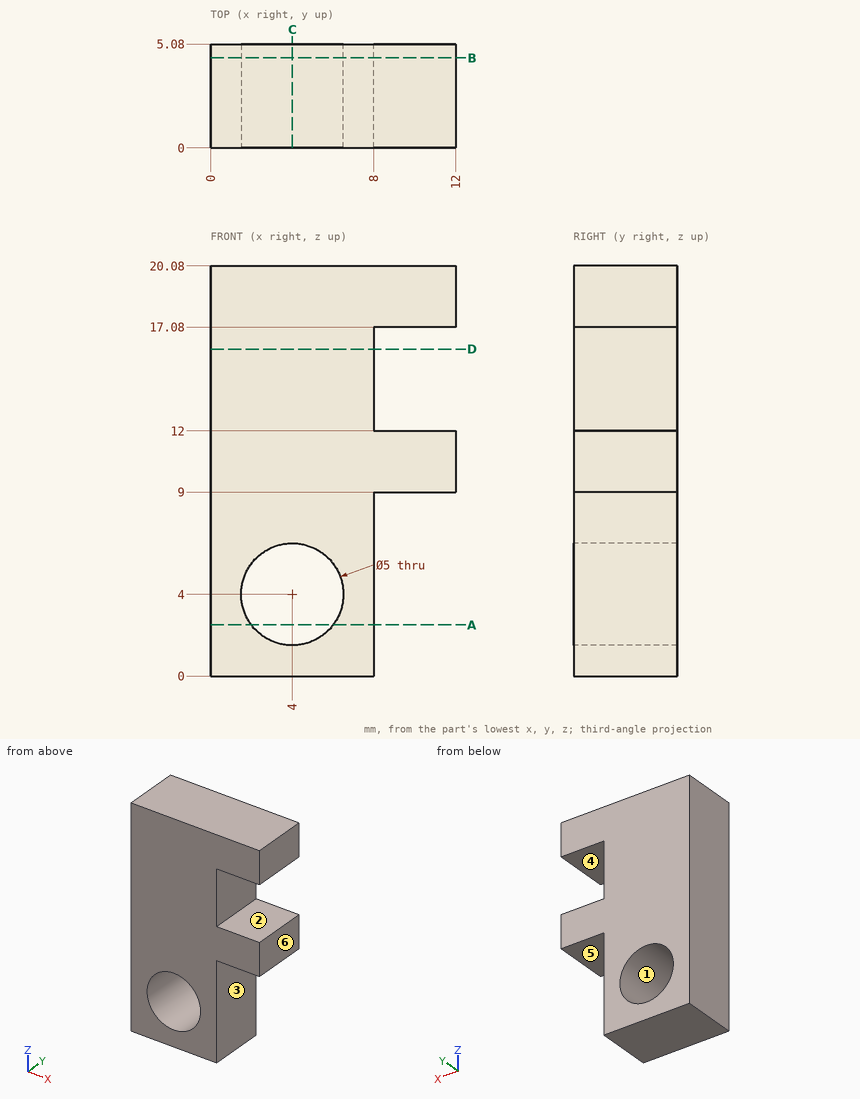
Could you check a few things on this drawing? It's one solid part, dimensions in mm from its lowest x, y, z. A direction names the side the tool comes from. Round coordinates to 2 decimals unless told otherwise and drop trailing zeros. Loops run counter-clockwise (first coordinate to the right, second up) from the corner with the lowest first, then second, coordinate; pieces in that order, holes last. Notation, with made-up numbers: (84.5, 76) -> (105.5, 76) arc R15 cw to (105.5, 101) -> close; hole circle Ø9 at (16.5, 40.25). An arc over 180 degrees is marked (long way). Answer as CSV lines item,"result".
1. If I drill on L1, parallel to Z at x = 4, y = 1.55; L2, parallel to X at y = 1.4, z = 4; L3, parallel to X at y = 4.4, z = 13.25, over which ranges is the centre line in solid material (lowest first)?
Final values:
L1,"z = 0 to 1.5, 6.5 to 20.08"
L2,"x = 0 to 1.5, 6.5 to 8"
L3,"x = 0 to 8"
2. If we section it at A-A on z = 2.5: Please give me the cut outline in (x, y).
Final values:
outline,"(0, 0) -> (2, 0) -> (2, 5.08) -> (0, 5.08) -> close; (6, 0) -> (8, 0) -> (8, 5.08) -> (6, 5.08) -> close"
3. If we section it at C-C on x = 4: Please give me the cut outline in (y, z), plus the area to 3 significant figures.
Final values:
outline,"(0, 0) -> (5.08, 0) -> (5.08, 1.5) -> (0, 1.5) -> close; (0, 6.5) -> (5.08, 6.5) -> (5.08, 20.08) -> (0, 20.08) -> close"
area,"76.6 mm^2"
4. Which directions (+Z, -Z, +X, -X, +Y, -Y) give clear straight access to the entire face, cutting with the end or side of a thin tool? Please do the marked faces 1, 2 and 3.
Final values:
face 1,"+Y, -Y"
face 2,"+X, +Y, -Y"
face 3,"-Z, +X, +Y, -Y"
5. If we section it at D-D on z = 16: Please give me the cut outline in (x, y).
Final values:
outline,"(0, 0) -> (8, 0) -> (8, 5.08) -> (0, 5.08) -> close"
6. For pin 1 (1 mm diameter, centred on y = 3, z = 16, fed in from +X); pin 2 (3 mm diameter, centred on x = 10.5, y = 1.5, fed in from -Z), each with a flat end and sliding along its axis, tell me the tip position at first contact or that it passes through.
Final values:
pin 1,"stops at x = 8"
pin 2,"stops at z = 9"
7. Thinking about a two-plate mould opening in Z: for the marked faces 4, 5 and 6, which applies, released by +Z, released by -Z, zero draft, split by the parting line, or undercut?
Final values:
face 4,"undercut"
face 5,"released by -Z"
face 6,"zero draft"
8. If we section it at B-B on y = 4.4: Please give me the cut outline in (x, z), plus the area to 3 significant figures.
Final values:
outline,"(0, 0) -> (8, 0) -> (8, 9) -> (12, 9) -> (12, 12) -> (8, 12) -> (8, 17.08) -> (12, 17.08) -> (12, 20.08) -> (0, 20.08) -> close; hole circle Ø5 at (4, 4)"
area,"165 mm^2"
